Input: part model. Units: mm. Frame: model coordinates. Face numbers are marked on the shaded views. A direction names the side the tool comes from. Round coordinates to 2 decimals unless told otherwise and drop trailing zeros. Loops run counter-clockwise (first coordinate to the right, second up) from the corner with the lowest first, then second, coordinate; pieces in that order, holes last. Notation, with made-up numbers: (-18.5, 58) - (35.5, 58) arc R13 ccw to (35.5, 73) - close; hole circle Ø1 at (39, 77). An arc over 180 degrees is marked (long way). One line per question, with ' | ' between items. Start each with the question number.
Item 1: Section B-B, the plane z = -7.5. Return loops of the section in (x, y), plus the area to 3 significant figures.
Item 2: Section D-D, the plane x = 20. Return loops of the section in (y, z), plus the area to 3 significant figures.
Item 3: Draft query along Z for the marked faces 4, 5 and 6. Return one class per face: pulls with the +Z half, pulls with the -Z half, needs draft (parallel to the pull), parting line crosses it, or undercut.
Item 4: First-contact query: pin 1 (7.5 mm diameter, centred on x = 48.5, z = -31, fed in from +Y); pin 2 (1.5 mm diameter, centred on y = 8.5, z = -30, fed in from +X); pin 3 (1.5 mm diameter, centred on y = 7, z = -48.5, fed in from -X). Flat tips, straight axial feed; report the tip coordinate or a pass-through.
Item 5: Section A-A, the plane x = 36. Return loops of the section in (y, z).
Item 6: Material intervals for line 1 along Z through (x, y) = (51.5, 2.15); line 2 along X through (y, z) = (1.1, -43.5); line 3 along X through (y, z) = (6.25, -35.5), sorted ascending.
Item 7: Set-up query: the marked faces 1, 2 and 3. Return all of +Z, -Z, +X, -X, +Y, -Y with unobstructed straight access to the full face (end or side cutting, diameter ignored); none if empty.
Item 8: Section C-C, the plane y = 2.25. Give the number of separate pieces and of enclosed holes in the cut face, plus the area to 3 significant figures.
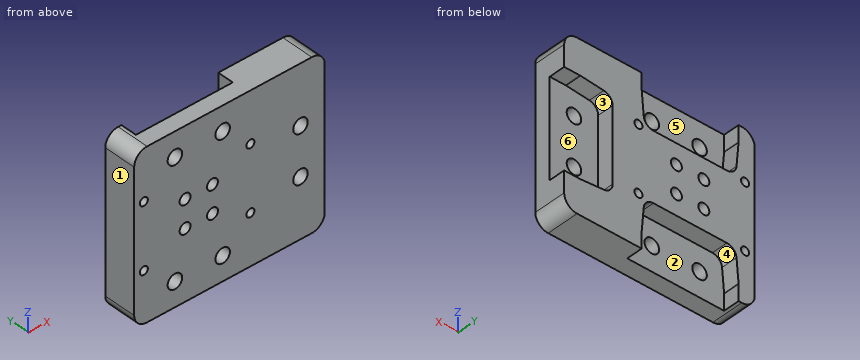
```python
from build123d import *

# Parameters (mm, degrees)
SKETCH_1_W          = 59
SKETCH_1_H          = 51
EXTRUDE_1_DEPTH     = 10
CUT_EXTRUDE_5_DEPTH = 5
HOLE_WIZARD_M31_D   = 3.4
FILLET_1_R          = 4
FILLET_2_R          = 4
CUT_EXTRUDE_6_DEPTH = 5
HOLE_WIZARD_M42_D   = 4.5
M3X0_51_D           = 2.5


with BuildPart() as part:
    # Эскиз1 → Бобышка-Вытянуть1 (new body)
    with BuildSketch(Plane(origin=(0, 0, 0), x_dir=(1, 0, 0), z_dir=(0, 1, 0))):
        with Locations((29.5, 25.5)):
            Rectangle(SKETCH_1_W, SKETCH_1_H)
    extrude(amount=EXTRUDE_1_DEPTH)

    # Эскиз13 → Вырез-Вытянуть5 (cut)
    with BuildSketch(Plane(origin=(28.521351565, 10, -17.681729678), x_dir=(1, 0, 0), z_dir=(0, 1, 0))):
        with BuildLine():
            Line((30.478648435, 22.818270322), (25.609631264, 22.818270322))
            ThreePointArc((25.609631264, 22.818270322), (25.478773101, 22.815414987), (25.348164035, 22.806854417))
            Line((25.348164035, 22.806854417), (18.217181207, 22.182974259))
            ThreePointArc((18.217181207, 22.182974259), (16.266816424, 21.221160788), (15.478648435, 19.194390165))
            Line((15.478648435, 19.194390165), (15.478648435, -3.55784952))
            ThreePointArc((15.478648435, -3.55784952), (16.266816424, -5.584620143), (18.217181207, -6.546433615))
            Line((18.217181207, -6.546433615), (25.348164035, -7.170313772))
            ThreePointArc((25.348164035, -7.170313772), (25.478773101, -7.178874342), (25.609631264, -7.181729678))
            Line((25.609631264, -7.181729678), (30.478648435, -7.181729678))
            Line((30.478648435, -7.181729678), (30.478648435, 22.818270322))
        make_face()
    extrude(amount=-CUT_EXTRUDE_5_DEPTH, mode=Mode.SUBTRACT)

    # Отверстие с зазором M31 (through all)
    with Locations(Plane(origin=(0, 0, 0), x_dir=(-1, 0, 0), z_dir=(0, -1, 0))):
        with Locations((-24.242640687, 29.742640687), (-15.757359313, 29.742640687), (-15.757359313, 21.257359313), (-24.242640687, 21.257359313)):
            Hole(HOLE_WIZARD_M31_D / 2)

    # Скругление1
    fillet_1_edges = [part.edges().sort_by_distance(p)[0] for p in [
        (0, 5, -51),
        (0, 5, 0),
    ]]
    fillet(fillet_1_edges, radius=FILLET_1_R)

    # Скругление2
    fillet_2_edges = [part.edges().sort_by_distance(p)[0] for p in [
        (59, 5, -51),
        (59, 5, 0),
    ]]
    fillet(fillet_2_edges, radius=FILLET_2_R)

    # Эскиз14 → Вырез-Вытянуть6 (cut)
    with BuildSketch(Plane(origin=(28.521351565, 10, -17.681729678), x_dir=(1, 0, 0), z_dir=(0, 1, 0))):
        with BuildLine():
            Line((-23.521351565, -12.812712506), (-23.521351565, -17.681729678))
            Line((-23.521351565, -17.681729678), (6.478648435, -17.681729678))
            Line((6.478648435, -17.681729678), (6.478648435, -12.812712506))
            ThreePointArc((6.478648435, -12.812712506), (6.4757931, -12.681854344), (6.467232529, -12.551245278))
            Line((6.467232529, -12.551245278), (5.843352372, -5.420262449))
            ThreePointArc((5.843352372, -5.420262449), (4.8815389, -3.469897667), (2.854768277, -2.681729678))
            Line((2.854768277, -2.681729678), (-19.897471408, -2.681729678))
            ThreePointArc((-19.897471408, -2.681729678), (-21.924242031, -3.469897667), (-22.886055502, -5.420262449))
            Line((-22.886055502, -5.420262449), (-23.509935659, -12.551245278))
            ThreePointArc((-23.509935659, -12.551245278), (-23.51849623, -12.681854344), (-23.521351565, -12.812712506))
        make_face()
        with BuildLine():
            Line((6.478648435, 28.449253151), (6.478648435, 33.318270322))
            Line((6.478648435, 33.318270322), (-23.521351565, 33.318270322))
            Line((-23.521351565, 33.318270322), (-23.521351565, 28.449253151))
            ThreePointArc((-23.521351565, 28.449253151), (-23.51849623, 28.318394989), (-23.509935659, 28.187785923))
            Line((-23.509935659, 28.187785923), (-22.886055502, 21.056803094))
            ThreePointArc((-22.886055502, 21.056803094), (-21.924242031, 19.106438312), (-19.897471408, 18.318270322))
            Line((-19.897471408, 18.318270322), (2.854768277, 18.318270322))
            ThreePointArc((2.854768277, 18.318270322), (4.8815389, 19.106438312), (5.843352372, 21.056803094))
            Line((5.843352372, 21.056803094), (6.467232529, 28.187785923))
            ThreePointArc((6.467232529, 28.187785923), (6.4757931, 28.318394989), (6.478648435, 28.449253151))
        make_face()
    extrude(amount=-CUT_EXTRUDE_6_DEPTH, mode=Mode.SUBTRACT)

    # Отверстие с зазором M42 (through all)
    with Locations(Plane(origin=(28.521351565, 5, -17.681729678), x_dir=(1, 0, 0), z_dir=(0, 1, 0))):
        with Locations((-15.911990736, 25.818270322), (-1.130712395, 25.818270322), (22.978648435, 15.208909493), (22.978648435, 0.427631152), (-1.130712395, -10.181729678), (-15.911990736, -10.181729678)):
            Hole(HOLE_WIZARD_M42_D / 2)

    # Отверстие обработанное метчиком M3x0.51 (through all)
    with Locations(Plane(origin=(33.500358967, 0, -26.410335717), x_dir=(-1, 0, 0), z_dir=(0, -1, 0))):
        with Locations((30.500358967, -10.910335717), (-2.499641033, -10.910335717), (-2.499641033, 9.089664283), (30.500358967, 9.089664283)):
            Hole(M3X0_51_D / 2)


solid = part.part
```
Return value:
1) outline: (0, 0) - (10.36, 0) - (10.36, 5) - (5.22, 5) - (5.22, 10) - (0, 10) - close; (14.86, 0) - (25.14, 0) - (25.14, 5) - (14.86, 5) - close; (29.64, 0) - (59, 0) - (59, 10) - (34.78, 10) - (34.78, 5) - (29.64, 5) - close | area: 397 mm2
2) outline: (0, -51) - (5, -51) - (5, -36) - (10, -36) - (10, -15) - (5, -15) - (5, 0) - (0, 0) - close | area: 360 mm2
3) face 4: pulls with the -Z half | face 5: needs draft | face 6: undercut
4) pin 1: y = 5 | pin 2: x = 44 | pin 3: x = 0.07
5) outline: (0, -51) - (10, -51) - (10, -36.75) - (0, -36.75) - close; (0, -34.25) - (10, -34.25) - (10, -16.75) - (0, -16.75) - close; (0, -14.25) - (10, -14.25) - (10, 0) - (0, 0) - close
6) line 1: -51 to -35.14, -30.64 to -20.36, -15.86 to 0 | line 2: 0 to 10.36, 14.86 to 25.14, 29.64 to 59 | line 3: 0 to 1.75, 4.25 to 34.75, 37.25 to 44
7) face 1: +Z, -Z, -X, +Y, -Y | face 2: -Z, +Y | face 3: +X, +Y
8) separate pieces: 1 | enclosed holes: 14 | area: 2,840 mm2
